Read the model definition and answer for the solid it produces. Units are mm, in the model's axes. Face numbers are marked on the shaded views. Give positions to 0.01 mm unless a question says otherwise; leave off trailing zeros. Order: outer loops, then holes, each group sorted by start corner. A loop starts at its lowest first (then second) coordinate and runs counter-clockwise, first axis right, second up. Notation, with made-up numbers: (51, 27) - (63, 27) arc R22 ccw to (63, 56) - close; hole circle Ø11 at (-4, 33.25). An arc over 180 degrees is marked (long way). Write each question's results on one line, items separated by ' | '. Start each with the question number.
Q1. Flat-ended cylindrical pins translate along their axes: P1, Ø1.8, axis at x = 0, z = 15, coming from the -Y side; P2, Ø3, axis at x = 59, z = 14, coming from the +Y side; P3, Ø1.8, axis at x = -1, z = 12, coming from the +Y side; P4, Ø1.5, axis at x = 36.5, z = 11, coming from the -Y side. Find the tip coordinate at first contact, or state that the pin passes through.
Q2. Find section D-D on x = -34.5. Give the vertices of the cut face in (y, z), and give its area (3 significant figures).
Q3. Find section A-A on y = 0. Give the vertices of the cut face in (x, z), and give its area (3 significant figures).
Q4. Find section C-C on y = -15.5. Give the vertices of the cut face in (x, z), and give its area (3 significant figures).
Q5. For a pull along X with two mould halves and no side action, classify the marked faces 1 and 2 as +X half, -X half, draft (parallel to the pull), parting line (faces both ways), or undercut.
Q6. Find the intervals of material crossed by line 1 along Y through (x, z) = (0, -2.9); line 2 along X through (y, z) = (-2, -4.25); line 3 along Z through (x, y) = (14, -68), in increasing order. Write a range as from..to.
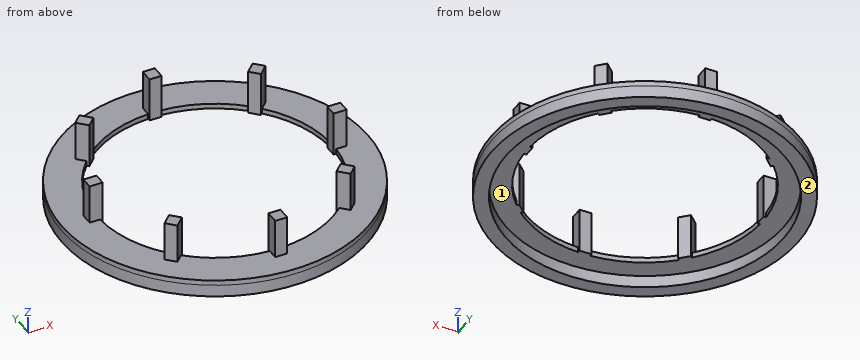
from build123d import *

# Parameters (mm, degrees)
F0_R     = 74.8284
F0_R_2   = 67.8942
F1_DEPTH = 5.969
F2_R     = 74.8284
F2_R_2   = 57.8104
F3_DEPTH = 2.54
F4_W     = 6.424342
F4_H     = 5.888975
F4_W_2   = 5.888975
F4_H_2   = 6.424342
F5_DEPTH = 21.8694


with BuildPart() as f1:
    # F0 (on Top) → F1 (new body)
    with BuildSketch(Plane.XY):
        Circle(F0_R)
        Circle(F0_R_2, mode=Mode.SUBTRACT)
    extrude(amount=-F1_DEPTH)

    # F2 (on Top) → F3 (join)
    with BuildSketch(Plane.XY):
        Circle(F2_R)
        Circle(F2_R_2, mode=Mode.SUBTRACT)
    extrude(amount=F3_DEPTH)

    # F4 (on Top) → F5 (join)
    with BuildSketch(Plane.XY):
        with Locations((-59.654696, 0.23042)):
            Rectangle(F4_W, F4_H)
        Polygon((-42.155891, -37.665894), (-46.698586, -42.208589), (-42.534452, -46.372723), (-37.991757, -41.830028), align=None)
        with Locations((-0.23042, -59.654696)):
            Rectangle(F4_W_2, F4_H_2)
        Polygon((37.665894, -42.155891), (42.208589, -46.698586), (46.372723, -42.534452), (41.830028, -37.991757), align=None)
        with Locations((59.654696, -0.23042)):
            Rectangle(F4_W, F4_H)
        Polygon((42.155891, 37.665894), (46.698586, 42.208589), (42.534452, 46.372723), (37.991757, 41.830028), align=None)
        with Locations((0.23042, 59.654696)):
            Rectangle(F4_W_2, F4_H_2)
        Polygon((-37.665894, 42.155891), (-42.208589, 46.698586), (-46.372723, 42.534452), (-41.830028, 37.991757), align=None)
    extrude(amount=F5_DEPTH)


solid = f1.part
Working result:
1) P1: y = -62.87 | P2: y = 2.71 | P3: y = 62.87 | P4: through
2) outline: (-66.4, -5.97) - (-58.48, -5.97) - (-58.48, 0) - (-46.39, 0) - (-46.39, 2.54) - (-66.4, 2.54) - close; (46.39, 0) - (58.48, 0) - (58.48, -5.97) - (66.4, -5.97) - (66.4, 2.54) - (46.39, 2.54) - close | area: 196 mm²
3) outline: (-74.83, -5.97) - (-67.89, -5.97) - (-67.89, 0) - (-56.44, 0) - (-56.44, 21.87) - (-62.87, 21.87) - (-62.87, 2.54) - (-74.83, 2.54) - close; (56.44, 0) - (67.89, 0) - (67.89, -5.97) - (74.83, -5.97) - (74.83, 2.54) - (62.87, 2.54) - (62.87, 21.87) - (56.44, 21.87) - close | area: 425 mm²
4) outline: (-73.21, -5.97) - (-66.1, -5.97) - (-66.1, 0) - (-55.69, 0) - (-55.69, 2.54) - (-73.21, 2.54) - close; (55.69, 0) - (66.1, 0) - (66.1, -5.97) - (73.21, -5.97) - (73.21, 2.54) - (55.69, 2.54) - close | area: 174 mm²
5) face 1: undercut | face 2: draft
6) line 1: -74.83..-67.89, 67.89..74.83 | line 2: -74.8..-67.86, 67.86..74.8 | line 3: -5.97..2.54
